```python
from build123d import *

# Parameters (mm, degrees)
SKETCH1_R                = 45
BOSS_EXTRUDE1_DEPTH      = 135
SKETCH2_R                = 35
CUT_EXTRUDE1_DEPTH       = 90
SKETCH3_R                = 37.5
SKETCH3_R_2              = 35
CUT_EXTRUDE2_DEPTH       = 25
SKETCH4_R                = 37.5
SKETCH4_R_2              = 35
CUT_EXTRUDE3_DEPTH       = 25
SKETCH5_R                = 7.5
CUT_EXTRUDE4_DEPTH       = 5
BOSS_EXTRUDE2_DEPTH      = 2
BOSS_EXTRUDE2_DEPTH_BACK = 4
SKETCH6_W                = 19.05
SKETCH6_H                = 25.4


with BuildPart() as part:
    # Sketch1 → Boss-Extrude1 (new body)
    with BuildSketch(Plane(origin=(0, 0, 0), x_dir=(1, 0, 0), z_dir=(0, 1, 0))):
        with Locations(Location((0, 0, 0), (0, 0, 270))):
            Circle(SKETCH1_R)
    extrude(amount=BOSS_EXTRUDE1_DEPTH)

    # Sketch2 → Cut-Extrude1 (cut)
    with BuildSketch(Plane(origin=(0, 135, 0), x_dir=(1, 0, 0), z_dir=(0, 1, 0))):
        with Locations(Location((0, 0, 0), (0, 0, 270))):
            Circle(SKETCH2_R)
    extrude(amount=-CUT_EXTRUDE1_DEPTH, mode=Mode.SUBTRACT)

    # Sketch3 → Cut-Extrude2 (cut)
    with BuildSketch(Plane(origin=(0, 128, 0), x_dir=(1, 0, 0), z_dir=(0, 1, 0))):
        with Locations(Location((0, 0, 0), (0, 0, 270))):
            Circle(SKETCH3_R)
        with Locations(Location((0, 0, 0), (0, 0, 270))):
            Circle(SKETCH3_R_2, mode=Mode.SUBTRACT)
    extrude(amount=-CUT_EXTRUDE2_DEPTH, mode=Mode.SUBTRACT)

    # Sketch4 → Cut-Extrude3 (cut)
    with BuildSketch(Plane(origin=(0, 89, 0), x_dir=(1, 0, 0), z_dir=(0, 1, 0))):
        with Locations(Location((0, 0, 0), (0, 0, 270))):
            Circle(SKETCH4_R)
        with Locations(Location((0, 0, 0), (0, 0, 270))):
            Circle(SKETCH4_R_2, mode=Mode.SUBTRACT)
    extrude(amount=-CUT_EXTRUDE3_DEPTH, mode=Mode.SUBTRACT)

    # Sketch5 → Cut-Extrude4 (cut)
    with BuildSketch(Plane(origin=(0, 45, 0), x_dir=(1, 0, 0), z_dir=(0, 1, 0))):
        with Locations(Location((0, 0, 0), (0, 0, 270))):
            Circle(SKETCH5_R)
    extrude(amount=-CUT_EXTRUDE4_DEPTH, mode=Mode.SUBTRACT)

    # Sketch6 → Boss-Extrude2 (add, two sides: drawn at the far end of the back side and taken through both)
    with BuildSketch(Plane.XY.offset(45).offset(-BOSS_EXTRUDE2_DEPTH_BACK)):
        with Locations((0, 22.7)):
            Rectangle(SKETCH6_W, SKETCH6_H)
    extrude(amount=BOSS_EXTRUDE2_DEPTH + BOSS_EXTRUDE2_DEPTH_BACK)


solid = part.part
```
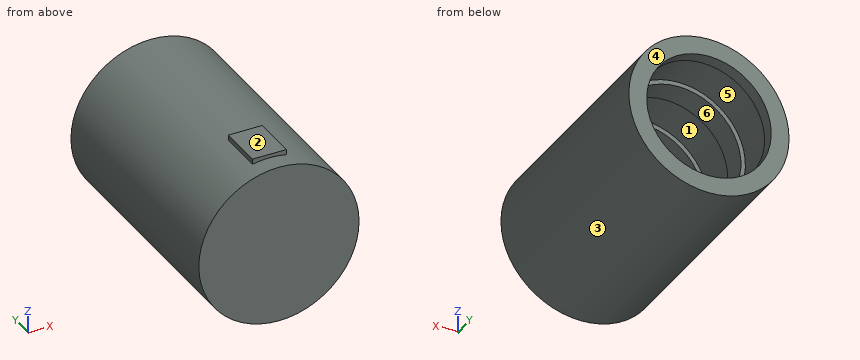
Part model, mm, in its own coordinate system. Face numbers are marked on the shaded views. A direction names the side the tool comes from. Round coordinates to 2 decimals unless told otherwise and drop trailing zeros. Order: outer loops, then holes, each group sorted by start corner. A loop starts at its lowest first (then second) coordinate and runs counter-clockwise, first axis right, second up. Notation, with made-up numbers: M 79,46 L 134,46 A24 ccw 134,85 Z; hole C -25.75,24 d6. An arc over 180 degrees is marked long. Put each result on its own line as item: value. Start each with the question number.
1. Tool access for the marked faces 1 and 2: list every direction of +Z, -Z, +X, -X, +Y, -Y with a clear straight run to the whole face (end or side of a thin tool).
2. Slice it at C-C on z = 0. List the corners of the cut face in (x, y), then the cut area to 4 significant figures.
3. Drill centre lines: probe 1 along X at (y, z) = (99, 0); probe 2 along X at (y, z) = (76.75, 0); probe 3 along Y at (x, z) = (-11, 22). Where is each one in solid material? Low to high. Write a range as [from, to].
4. Two-plate mould, pull along X, no slides. Class the marked faces 3, 4, 5 and 6: +X half, -X half, draft (parallel to the pull), parting line (faces both ways), or undercut.
5. Drop flat-ended pins along their axis: pin 1 (2.5 mm diameter, centred on y = 23.5, z = 46, fed in from -X) (3 decimals); pin 2 (12 mm diameter, centred on y = 49, z = 3.5, fed in from -X); pin 3 (4.5 mm diameter, centred on x = -1, z = 2.5, fed in from +Y). Give the stop position or say it passes through.
6. Slice it at B-B on y = 69. List the corners of the cut face in (x, z).
7. Slice it at D-D on y = 29. List the corners of the cut face in (x, z) (3 decimals), then the cut area to 3 significant figures.
Findings:
1. face 1: none
1. face 2: +Z, +X, -X, +Y, -Y
2. outline: M -45,0 L 45,0 L 45,135 L 35,135 L 35,128 L 37.5,128 L 37.5,103 L 35,103 L 35,89 L 37.5,89 L 37.5,64 L 35,64 L 35,45 L 7.5,45 L 7.5,40 L -7.5,40 L -7.5,45 L -35,45 L -35,64 L -37.5,64 L -37.5,89 L -35,89 L -35,103 L -37.5,103 L -37.5,128 L -35,128 L -35,135 L -45,135 Z
2. area: 5,525 mm2
3. probe 1: [-45, -35], [35, 45]
3. probe 2: [-45, -37.5], [37.5, 45]
3. probe 3: [0, 45]
4. face 3: parting line
4. face 4: draft
4. face 5: undercut
4. face 6: undercut
5. pin 1: x = -9.525
5. pin 2: x = -45
5. pin 3: y = 40
6. outline: C 0,0 d90; hole C 0,0 d75
7. outline: M -9.525,43.98 A45 ccw long 9.525,43.98 L 9.525,47 L -9.525,47 Z
7. area: 6,410 mm2
